Model file for the job. Use its own axes, mm. Round coordinates to 2 decimals unless told otherwise and drop trailing zeros. Order: outer loops, then holes, each group sorted by start corner. A loop starts at its lowest first (then second) coordinate and runs counter-clockwise, first axis right, second up. Notation, with made-up numbers: (63.25, 12.25) - (113.25, 12.25) arc R9 ccw to (113.25, 25.25) - close; hole circle Ø5 at (52, 29). An arc over 180 degrees is marked (long way). Use one line per item in the form item = value.
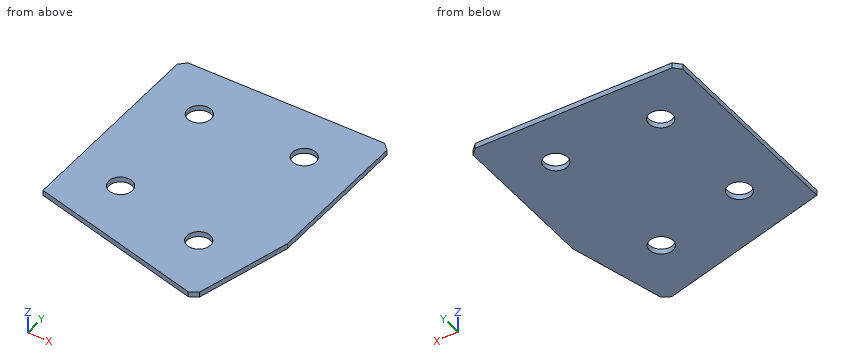
from build123d import *

# Parameters (mm, degrees)
EXTRUDE_1_DEPTH   = 2
HOLE_WIZARD_M81_D = 9
CHAMFER_1_SIZE    = 2.5


with BuildPart() as part:
    # Эскиз3 → Бобышка-Вытянуть1 (new body)
    with BuildSketch(Plane(origin=(0, 0, 0), x_dir=(1, 0, 0), z_dir=(0, 0, -1))):
        Polygon((0, 0), (80, 0), (80, 60.024888178), (69.647238196, 98.66192123), (0, 80), align=None)
    extrude(amount=EXTRUDE_1_DEPTH)

    # Отверстие с зазором M81 (through all)
    with Locations(Plane(origin=(0, 0, -2), x_dir=(1, 0, 0), z_dir=(0, 0, -1))):
        with Locations((20, 20), (60, 20), (19.318516526, 64.470857294), (55.505102572, 74.167023802)):
            Hole(HOLE_WIZARD_M81_D / 2)

    # Фаска1
    chamfer_1_edges = [part.edges().sort_by_distance(p)[0] for p in [
        (69.647238196, -98.66192123, -1),
        (80, 0, -1),
        (0, 0, -1),
    ]]
    chamfer(chamfer_1_edges, length=CHAMFER_1_SIZE)


solid = part.part
(1) Slice it at D-D on z = -1.35. Give the cut face in (x, y).
Report:
outline = (0, -80) - (67.23, -98.01) - (70.29, -96.25) - (80, -60.02) - (80, -2.5) - (77.5, 0) - (2.5, 0) - (0, -2.5) - close; hole circle Ø9 at (19.32, -64.47); hole circle Ø9 at (20, -20); hole circle Ø9 at (55.51, -74.17); hole circle Ø9 at (60, -20)
(2) Slice it at A-A on y = -20. Give the cut face in (x, z), then the cut area to 3 significant figures.
Report:
outline = (0, -2) - (15.5, -2) - (15.5, 0) - (0, 0) - close; (24.5, -2) - (55.5, -2) - (55.5, 0) - (24.5, 0) - close; (64.5, -2) - (80, -2) - (80, 0) - (64.5, 0) - close
area = 124 mm2
(3) Slice it at B-B on x = 20. Give the cut face in (y, z).
Report:
outline = (-85.36, -2) - (-68.92, -2) - (-68.92, 0) - (-85.36, 0) - close; (-60.02, -2) - (-24.5, -2) - (-24.5, 0) - (-60.02, 0) - close; (-15.5, -2) - (0, -2) - (0, 0) - (-15.5, 0) - close
(4) Probe probe 1 along X at (y, z) = (-20, -1.4); probe 2 along X at (y, z) = (-18.5, -0.35); probe 3 along X at (y, z) = (-70.5, -0.75). List the from-to ranges inside material, lowest first. Write a range as [from, to].
Report:
probe_1 = [0, 15.5], [24.5, 55.5], [64.5, 80]
probe_2 = [0, 15.76], [24.24, 55.76], [64.24, 80]
probe_3 = [0, 52.9], [58.11, 77.19]
(5) Slice it at C-C on y = -77. Give the cut face in (x, z), then the cut area to 3 significant figures.
Report:
outline = (0, -2) - (52.01, -2) - (52.01, 0) - (0, 0) - close; (59, -2) - (75.45, -2) - (75.45, 0) - (59, 0) - close
area = 137 mm2
